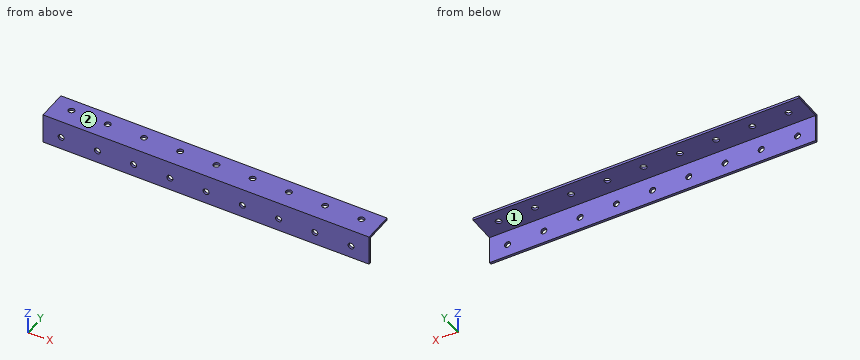
from build123d import *

# Parameters (mm, degrees)
EXTRUDE_1_DEPTH     = 540
SKETCH_2_R          = 5
CUT_EXTRUDE_1_DEPTH = 51
SKETCH_3_R          = 5
CUT_EXTRUDE_2_DEPTH = 51


with BuildPart() as part:
    # Эскиз1 → Вытянуть-Тонкостенный1 (new body)
    with BuildSketch(Plane(origin=(0, 0, 0), x_dir=(0, 0, -1), z_dir=(1, 0, 0))):
        Polygon((50, 0), (0, 0), (0, 50), (4, 50), (4, 4), (50, 4), align=None)
    extrude(amount=EXTRUDE_1_DEPTH)

    # Эскиз2 → Вырез-Вытянуть1 (cut, through all)
    with BuildSketch(Plane.XY):
        with Locations((30, 29)):
            Circle(SKETCH_2_R)
        with Locations((90, 29)):
            Circle(SKETCH_2_R)
        with Locations((150, 29)):
            Circle(SKETCH_2_R)
        with Locations((210, 29)):
            Circle(SKETCH_2_R)
        with Locations((270, 29)):
            Circle(SKETCH_2_R)
        with Locations((330, 29)):
            Circle(SKETCH_2_R)
        with Locations((390, 29)):
            Circle(SKETCH_2_R)
        with Locations((450, 29)):
            Circle(SKETCH_2_R)
        with Locations((510, 29)):
            Circle(SKETCH_2_R)
    extrude(amount=-CUT_EXTRUDE_1_DEPTH, mode=Mode.SUBTRACT)

    # Эскиз3 → Вырез-Вытянуть2 (cut, through all)
    with BuildSketch(Plane.XZ):
        with Locations((30, -29)):
            Circle(SKETCH_3_R)
        with Locations((90, -29)):
            Circle(SKETCH_3_R)
        with Locations((150, -29)):
            Circle(SKETCH_3_R)
        with Locations((210, -29)):
            Circle(SKETCH_3_R)
        with Locations((270, -29)):
            Circle(SKETCH_3_R)
        with Locations((330, -29)):
            Circle(SKETCH_3_R)
        with Locations((390, -29)):
            Circle(SKETCH_3_R)
        with Locations((450, -29)):
            Circle(SKETCH_3_R)
        with Locations((510, -29)):
            Circle(SKETCH_3_R)
    extrude(amount=-CUT_EXTRUDE_2_DEPTH, mode=Mode.SUBTRACT)


solid = part.part
Verification items for the finished model (mm, model axes). Face numbers are marked on the shaded views. A direction names the side the tool comes from. Give positions to 0.01 mm unless a question says otherwise; leave off trailing zeros. Write each loop counter-clockwise with the first axis right and the second up, starting at its lowest first coordinate (ties: lowest second). Pieces come first, ordered by that corner, then holes. Notation, with made-up numbers: (27.5, 84.5) - (81.5, 84.5) arc R31 ccw to (81.5, 116.5) - close; hole circle Ø11 at (29.25, 37.5). An arc over 180 degrees is marked (long way). Answer as CSV lines item,"result". Start each with the question number.
1. Sectioned sample at B-B (x = 371.5). Record the boundary of the cut face in (y, z), then the cut area to 3 significant figures.
2. Sectioned sample at C-C (y = 15). Record the boundary of the cut face in (x, z), then the cut area to 3 significant figures.
3. Sectioned sample at D-D (z = -16). Record the boundary of the cut face in (x, y), then the cut area to 3 significant figures.
4. Thickness scan on line 1 (Z direction, x = 390, y = 1); line 2 (Y direction, x = 216, z = -42); line 3 (Z direction, x = 209, y = 13). Record the ranges inside material, lowest first.
5. Depth check by flat-ended pin: pin 1 (9 mm diameter, centred on x = 150, y = 29, fed in from +Z); pin 2 (23 mm diameter, centred on x = 317.5, y = 22, fed in from -Z); pin 3 (16 mm diameter, centred on x = 270, z = -29, fed in from +Y). Enter the tip coordinate at first touch or a pass-through.
6. Set-up check for the marked faces 1 and 2: record each of +Z, -Z, +X, -X, +Y, -Y from which the full face is reachable in a straight line by a thin tool's end or side.
7. Sectioned sample at A-A (x = 30). Record the boundary of the cut face in (y, z), then the cut area to 3 significant figures.
Derived:
1,outline,"(0, -50) - (4, -50) - (4, -4) - (50, -4) - (50, 0) - (0, 0) - close"
1,area,"384 mm²"
2,outline,"(0, -4) - (540, -4) - (540, 0) - (0, 0) - close"
2,area,"2,160 mm²"
3,outline,"(0, 0) - (540, 0) - (540, 4) - (0, 4) - close"
3,area,"2,160 mm²"
4,line 1,"-50 to -34, -24 to 0"
4,line 2,"0 to 4"
4,line 3,"-4 to 0"
5,pin 1,"through"
5,pin 2,"z = -4"
5,pin 3,"y = 4"
6,face 1,"-Z, +X, -X, +Y"
6,face 2,"+Z, +X, -X, +Y, -Y"
7,outline,"(0, -50) - (4, -50) - (4, -34) - (0, -34) - close; (0, -24) - (4, -24) - (4, -4) - (24, -4) - (24, 0) - (0, 0) - close; (34, -4) - (50, -4) - (50, 0) - (34, 0) - close"
7,area,"304 mm²"
